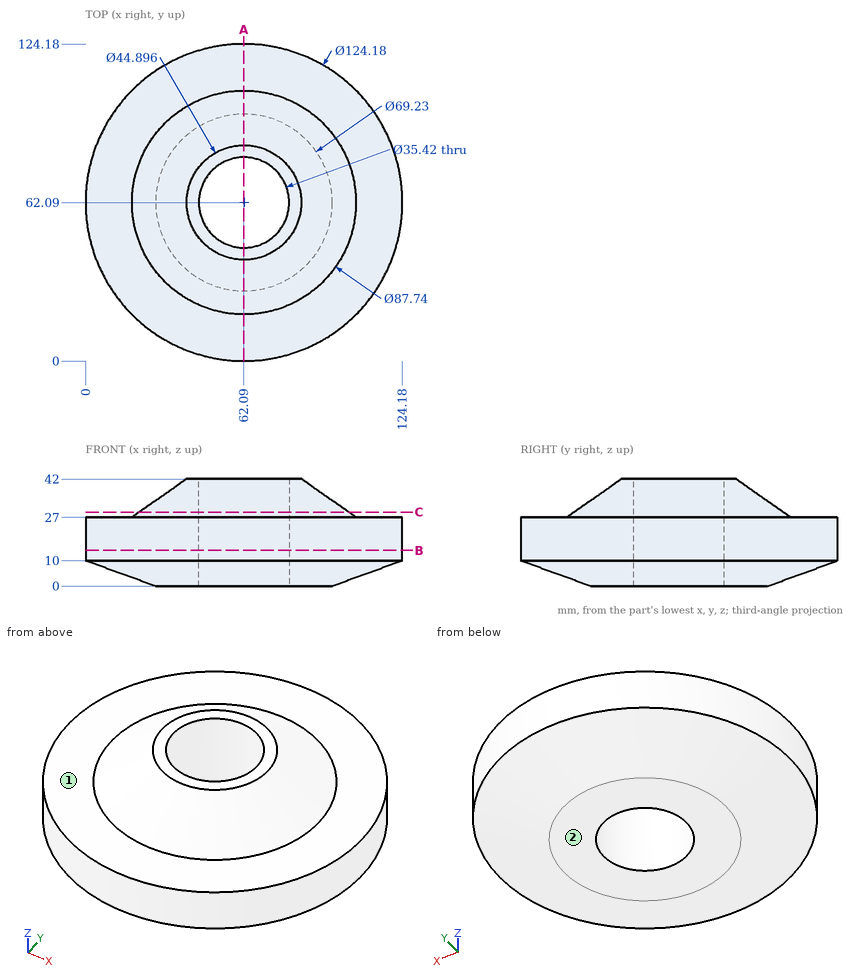
Print and shaded views of the part. All mm, measured from the part's lowest x, y and z. A direction names the side the tool comes from. Coordinates: 2 decimals unless noted, no trailing zeros. Order: outer loops, then holes, each group sorted by start corner. A loop starts at its lowest first (then second) coordinate and runs counter-clockwise, first axis right, second up. Notation, with made-up numbers: (-38, 88.25) - (-17, 88.25) arc R20 cw to (-17, 114.25) - close; hole circle Ø10 at (84.5, -21.5). An arc over 180 degrees is marked (long way). Return JSON: item names as keys, results as strings. Group by question number.
Item 1: Cut at C-C (z = 29). List the corners of the cut face in (x, y).
Item 2: Drill centre lines: probe 1 along Y at (x, z) = (62.09, 18.5); probe 2 along X at (y, z) = (62, 33); probe 3 along X at (y, z) = (57, 15). Where is each one in solid material? Low to high. Write a range as from..to.
Item 3: Cut at B-B (z = 14). List the corners of the cut face in (x, y), plus the area to 3 significant figures.
Item 4: Pin check, flat tips, straight feed: pin 1 (3 mm diameter, centred on x = 55, y = 17, fed in from +Z); pin 2 (4 mm diameter, centred on x = 110, y = 93.5, fed in from -Z) (1 decimal); pin 3 (12 mm diameter, centred on y = 34, z = 29.5, fed in from -X). Stop position of each tip, or through.
Item 5: Cut at A-A (x = 62.09). List the corners of the cut face in (y, z) (1 decimal).
Item 6: Which spindle directions (+Z, -Z, +X, -X, +Y, -Y) get a long thin tool onto all of the face, cutting with end or side? Do the marked faces 1 and 2. Say none if no direction does.
Check values:
{
 "1": {"outline": "circle Ø82.03 at (62.09, 62.09); hole circle Ø35.42 at (62.09, 62.09)"},
 "2": {"probe 1": "y = 0..44.38, 79.8..124.18", "probe 2": "x = 26.79..44.38, 79.8..97.39", "probe 3": "x = 0.21..45.13, 79.05..123.97"},
 "3": {"outline": "circle Ø124.18 at (62.09, 62.09); hole circle Ø35.42 at (62.09, 62.09)", "area": "11,100 mm2"},
 "4": {"pin 1": "stops at z = 27", "pin 2": "stops at z = 7.5", "pin 3": "stops at x = 4.27"},
 "5": {"outline": "(0, 10) - (27.5, 0) - (44.4, 0) - (44.4, 42) - (39.6, 42) - (18.2, 27) - (0, 27) - close; (79.8, 0) - (96.7, 0) - (124.2, 10) - (124.2, 27) - (106, 27) - (84.5, 42) - (79.8, 42) - close"},
 "6": {"face 1": "+Z", "face 2": "-Z, +X, -X, +Y, -Y"}
}
